Model file for the job. Use its own axes, mm. A direction names the side the tool comes from. Coordinates: 2 decimals unless noted, no trailing zeros. Write each loop counter-clockwise with the first axis right and the second up, starting at its lowest first coordinate (ties: lowest second). Pieces come first, ordered by that corner, then holes.
Q1. Pull direction Y, two halves, no side cores. Call faces 4 (the cylindrical face through (-17.456, 12.38, 4.275)), 5 (the flat face through (13, 11, 11.303)), 6 (the cylindrical face through (-5.276, 17.318, 10.402)): released by +Y, released by -Y, zero draft, split by the parting line, or undercut.
Q2. Which spindle directions (+Z, -Z, +X, -X, +Y, -Y) get a long thin tool onto all of the face, cutting with end or side? Do faces 1 (the cylindrical face through (6.073, 16.058, 4.157)), 2 (the flat face through (13, 19, 11.303)), 3 (the cylindrical face through (14.94, 17.86, 10.4)). Say none if no direction does.
Q3. Band-saw the part on C-C, the plane x = 17. Write the cut outline in (y, z) (3 decimals).
Q4. Pin check, flat tip, straight feed: P1, Ø2.5, axis at x = -22.5, y = 13.5, coming from the -Z side. Stop position of the tip, or through.
Q5. Band-saw the part on B-B, the plane x = -29. Write the cut outline in (y, z) (3 decimals), plus the area to 3 significant figures.
Q6. Band-saw the part on A-A, the plane z = 7.75. State how many separate pieces and enclosed holes the cut face has, plus the area to 3 significant figures.
Q7. Drill centre lines: probe 1 along Y at (x, z) = (7, 5.5); probe 2 along Y at (x, z) = (17, 1.5); probe 3 along X at (y, z) = (20.75, 7.5). Where is each one in solid material? Low to high.
from build123d import *

# Parameters (mm, degrees)
F0_W     = 64.1096
F0_H     = 15.875
F1_DEPTH = 9.525
F2_R     = 2.4257
F3_DEPTH = 1.778
F4_W     = 61.9252
F4_H     = 13.6906
F5_DEPTH = 8.4328
F6_R     = 3.2512
F6_R_2   = 3.401353
F7_DEPTH = 8.4328
F8_R     = 2.4638
F9_DEPTH = 8.4328


with BuildPart() as f1:
    # F0 (on Top) → F1 (new body)
    with BuildSketch(Plane.XY):
        with Locations((-7.36389, 14.818856)):
            Rectangle(F0_W, F0_H)
    extrude(amount=F1_DEPTH)

    # F2 (on face) → F3 (join)
    with BuildSketch(Plane.XY.offset(9.525)):
        with Locations((-35.45629, 18.793956)):
            Circle(F2_R)
        with Locations((-27.42989, 18.793956)):
            Circle(F2_R)
        with Locations((-19.40349, 18.793956)):
            Circle(F2_R)
        with Locations((-11.37709, 18.793956)):
            Circle(F2_R)
        with Locations((-3.35069, 18.793956)):
            Circle(F2_R)
        with Locations((4.67571, 18.793956)):
            Circle(F2_R)
        with Locations((12.70211, 18.793956)):
            Circle(F2_R)
        with Locations((20.72851, 18.793956)):
            Circle(F2_R)
        with Locations((-35.45629, 10.843756)):
            Circle(F2_R)
        with Locations((-27.42989, 10.843756)):
            Circle(F2_R)
        with Locations((-19.40349, 10.843756)):
            Circle(F2_R)
        with Locations((-11.37709, 10.843756)):
            Circle(F2_R)
        with Locations((-3.35069, 10.843756)):
            Circle(F2_R)
        with Locations((4.67571, 10.843756)):
            Circle(F2_R)
        with Locations((20.72851, 10.843756)):
            Circle(F2_R)
        with Locations((12.70211, 10.843756)):
            Circle(F2_R)
    extrude(amount=F3_DEPTH)

    # F4 (on face) → F5 (cut)
    with BuildSketch(Plane(origin=(0, 0, 0), x_dir=(1, 0, 0), z_dir=(0, 0, -1))):
        with Locations((-7.36389, -14.818856)):
            Rectangle(F4_W, F4_H)
    extrude(amount=-F5_DEPTH, mode=Mode.SUBTRACT)

    # F6 (on face) → F7 (join)
    with BuildSketch(Plane(origin=(0, 0, 8.4328), x_dir=(1, 0, 0), z_dir=(0, 0, -1))):
        with Locations((-30.45249, -14.577556)):
            Circle(F6_R)
        with Locations((15.72471, -14.577556)):
            Circle(F6_R_2)
        with Locations((-22.75629, -14.577556)):
            Circle(F6_R)
        with Locations((-15.06009, -14.577556)):
            Circle(F6_R)
        with Locations((-7.36389, -14.577556)):
            Circle(F6_R)
        with Locations((0.33231, -14.577556)):
            Circle(F6_R)
        with Locations((8.02851, -14.558641)):
            Circle(F6_R)
    extrude(amount=F7_DEPTH)

    # F8 (on face) → F9 (cut)
    with BuildSketch(Plane(origin=(0, 0, 0), x_dir=(1, 0, 0), z_dir=(0, 0, -1))):
        with Locations((-30.45249, -14.577556)):
            Circle(F8_R)
        with Locations((-22.75629, -14.577556)):
            Circle(F8_R)
        with Locations((-15.06009, -14.577556)):
            Circle(F8_R)
        with Locations((-7.36389, -14.577556)):
            Circle(F8_R)
        with Locations((0.33231, -14.577556)):
            Circle(F8_R)
        with Locations((8.02851, -14.558641)):
            Circle(F8_R)
        with Locations((15.72471, -14.577556)):
            Circle(F8_R)
    extrude(amount=-F9_DEPTH, mode=Mode.SUBTRACT)


solid = f1.part
Answer sheet:
1. face 4: undercut
1. face 5: zero draft
1. face 6: undercut
2. face 1: -Z
2. face 2: +Z, +X, -X, +Y, -Y
2. face 3: +Z
3. outline: (6.881, 0) - (7.974, 0) - (7.974, 8.433) - (11.424, 8.433) - (11.424, 0) - (12.469, 0) - (12.469, 8.433) - (16.686, 8.433) - (16.686, 0) - (17.731, 0) - (17.731, 8.433) - (21.664, 8.433) - (21.664, 0) - (22.756, 0) - (22.756, 9.525) - (6.881, 9.525) - close
4. P1: stops at z = 8.43
5. outline: (6.881, 0) - (7.974, 0) - (7.974, 8.433) - (11.669, 8.433) - (11.669, 0) - (12.587, 0) - (12.587, 8.433) - (16.568, 8.433) - (16.568, 0) - (17.486, 0) - (17.486, 8.433) - (21.664, 8.433) - (21.664, 0) - (22.756, 0) - (22.756, 9.525) - (20.643, 9.525) - (20.643, 11.303) - (16.945, 11.303) - (16.945, 9.525) - (12.693, 9.525) - (12.693, 11.303) - (8.995, 11.303) - (8.995, 9.525) - (6.881, 9.525) - close
5. area: 64.4 mm2
6. separate pieces: 8
6. enclosed holes: 8
6. area: 272 mm2
7. probe 1: y = 6.88 to 7.97, 11.47 to 12.32, 16.8 to 17.64, 21.66 to 22.76
7. probe 2: y = 6.88 to 7.97, 11.42 to 12.47, 16.69 to 17.73, 21.66 to 22.76
7. probe 3: x = -39.42 to -38.33, 23.6 to 24.69
